Read the model definition and answer for the solid it produces. Units are mm, in the model's axes. A direction names the side the tool comes from. Give positions to 0.01 mm unless a question says otherwise; leave off trailing zeros. Order: outer loops, then holes, each group sorted by start corner. A loop starts at its lowest first (then second) coordinate and runs counter-clockwise, first axis right, second up. Notation, with made-up numbers: (8, 71) - (44, 71) arc R33 cw to (44, 108) - close; hole circle Ø11 at (80, -24.5). An arc over 180 degrees is marked (long way). Use a Markdown table: item, result. Add a question column.
1. Flat-ended cylindrical pins translate along their axes: P1, Ø3.5, axis at x = 16.87, y = 14, coming from the -Z side; P2, Ø10, axis at y = 16, z = 8, coming from the +X side; P3, Ø9, axis at x = 18.5, y = 14.5, coming from the +Z side; P4, Ø3, axis at y = 8.5, z = 9.5, coming from the -X side. Find the tip coordinate at first contact, or state that the pin passes through.
2. Which of the six approach directions +Z, -Z, +X, -X, +Y, -Y give full straight-line access (tool end or side, diameter ignored) to faces 4 (the flat face through (-9, 14, 12.988)), 5 (the flat face through (-19.4, 13.8, -10)), 6 (the flat face through (10, 14, 3))?
3. For a pull along Z with two mould halves and no side action, classify faces 1 (the flat face through (1.021, 14, 12)), 2 (the cylindrical face through (-0.326, 12.325, -7.743)), 3 (the cylindrical face through (10.86, 14.2, -9.1)) as released by +Z, released by -Z, zero draft, split by the parting line, or undercut.
4. A cutting plane is placed at C-C on y = 14. State how many separate pieces and enclosed holes the cut face has, and give its area (3 significant figures).
5. A cutting plane is placed at A-A on x = 6. Determine the outline of the cut face in (y, z), and give its area (3 significant figures).
6. A cutting plane is placed at B-B on z = 0. Determine the outline of the cut face in (x, y).
7. A cutting plane is placed at D-D on x = -5.5. Determine the outline of the cut face in (y, z).
8. Consider L1, parallel to X at y = 16.5, z = 0; L2, parallel to X at y = 26.3, z = 0; L3, parallel to Z at x = -22.5, y = 14. Determine where each line is inside the solid, lowest interval first.
```python
from build123d import *

# Parameters (mm, degrees)
BOSS_EXTRUDE1_DEPTH = 28
SKETCH2_R           = 1.5
CUT_EXTRUDE1_DEPTH  = 20
CUT_EXTRUDE2_DEPTH  = 2
SKETCH4_R           = 2
CUT_EXTRUDE3_DEPTH  = 3
FILLET1_R           = 3
FILLET2_R           = 3
SKETCH5_R           = 7.75
CUT_EXTRUDE4_DEPTH  = 25


with BuildPart() as part:
    # Sketch1 → Boss-Extrude1 (new body)
    with BuildSketch(Plane(origin=(0, 0, 0), x_dir=(1, 0, 0), z_dir=(0, 1, 0))):
        with BuildLine():
            Line((-25.631117397, 10), (-10, 10))
            Line((-10, 10), (-10, -13.238049007))
            Line((-10, -13.238049007), (-1.021428571, -13.238049007))
            Line((-1.021428571, -13.238049007), (-1.021428571, -7.076664728))
            ThreePointArc((-1.021428571, -7.076664728), (0, 7.15), (1.021428571, -7.076664728))
            Line((1.021428571, -7.076664728), (1.021428571, -13.238049007))
            Line((1.021428571, -13.238049007), (10, -13.238049007))
            Line((10, -13.238049007), (10, 10))
            Line((10, 10), (24.368882603, 10))
            Line((24.368882603, 10), (24.368882603, 13))
            Line((24.368882603, 13), (-25.631117397, 13))
            Line((-25.631117397, 13), (-25.631117397, 10))
        make_face()
    extrude(amount=BOSS_EXTRUDE1_DEPTH)

    # Sketch2 → Cut-Extrude1 (cut)
    with BuildSketch(Plane.ZY.offset(10)):
        with Locations((10.238049007, 14)):
            Circle(SKETCH2_R)
    extrude(amount=-CUT_EXTRUDE1_DEPTH, mode=Mode.SUBTRACT)

    # Sketch3 → Cut-Extrude2 (cut)
    with BuildSketch(Plane.ZY.offset(10)):
        Polygon((10.238049007, 17.175426481), (7.488049007, 15.58771324), (7.488049007, 12.41228676), (10.238049007, 10.824573519), (12.988049007, 12.41228676), (12.988049007, 15.58771324), align=None)
    extrude(amount=-CUT_EXTRUDE2_DEPTH, mode=Mode.SUBTRACT)

    # Sketch4 → Cut-Extrude3 (cut)
    with BuildSketch(Plane(origin=(0, 0, -13), x_dir=(-1, 0, 0), z_dir=(0, 0, -1))):
        with Locations((-16.868882603, 14)):
            Circle(SKETCH4_R)
        with Locations(Location((16.868882603, 14, 0), (0, 0, 180))):
            Circle(SKETCH4_R)
    extrude(amount=-CUT_EXTRUDE3_DEPTH, mode=Mode.SUBTRACT)

    # Fillet1
    fillet1_edges = [part.edges().sort_by_distance(p)[0] for p in [
        (10, 14, -10),
    ]]
    fillet(fillet1_edges, radius=FILLET1_R)

    # Fillet2
    fillet2_edges = [part.edges().sort_by_distance(p)[0] for p in [
        (-10, 14, -10),
    ]]
    fillet(fillet2_edges, radius=FILLET2_R)

    # Sketch5 → Cut-Extrude4 (cut)
    with BuildSketch(Plane.XZ):
        Circle(SKETCH5_R)
    extrude(amount=-CUT_EXTRUDE4_DEPTH, mode=Mode.SUBTRACT)


solid = part.part
```
Output values:
| question | item | result |
|---|---|---|
| 1 | P1 | through |
| 1 | P2 | x = 10 |
| 1 | P3 | z = -10 |
| 1 | P4 | x = -10 |
| 2 | face 4 | -X |
| 2 | face 5 | +Z, -X, +Y, -Y |
| 2 | face 6 | +Z, +X, +Y, -Y |
| 3 | face 1 | zero draft |
| 3 | face 2 | undercut |
| 3 | face 3 | released by +Z |
| 4 | separate pieces | 5 |
| 4 | enclosed holes | 0 |
| 4 | area | 336 mm² |
| 5 | outline | (0, -13) - (28, -13) - (28, -3.89) - (25, -3.89) - (25, -4.91) - (0, -4.91) - close; (0, 4.91) - (25, 4.91) - (25, 3.89) - (28, 3.89) - (28, 13.24) - (0, 13.24) - close; hole circle Ø3 at (14, 10.24) |
| 5 | area | 459 mm² |
| 6 | outline | (-10, 0) - (-7.75, 0) - (-7.75, 25) - (-7.15, 25) - (-7.15, 28) - (-10, 28) - close; (7.15, 25) - (7.75, 25) - (7.75, 0) - (10, 0) - (10, 28) - (7.15, 28) - close |
| 7 | outline | (0, -13) - (28, -13) - (28, -4.57) - (25, -4.57) - (25, -5.46) - (0, -5.46) - close; (0, 5.46) - (25, 5.46) - (25, 4.57) - (28, 4.57) - (28, 13.24) - (0, 13.24) - close; hole circle Ø3 at (14, 10.24) |
| 8 | L1 | -10 to -7.75, 7.75 to 10 |
| 8 | L2 | -10 to -7.15, 7.15 to 10 |
| 8 | L3 | -13 to -10 |
